Part model, mm, in its own coordinate system. A direction names the side the tool comes from. Give positions to 0.01 mm unless a question says otherwise; leave off trailing zeros. Order: outer loops, then holes, each group sorted by start corner. A loop starts at its lowest first (then second) coordinate and runs counter-clockwise, first axis right, second up. Notation, with made-up numbers: (85.5, 54) - (123.5, 54) arc R20 ccw to (123.5, 73) - close; hole circle Ø3 at (5.25, 41.25). An arc over 180 degrees is marked (long way). Use a Markdown table: item, result. Add a question column.
from build123d import *

# Parameters (mm, degrees)
BOSS_EXTRUDE1_DEPTH = 129


with BuildPart() as part:
    # Sketch1 → Boss-Extrude1 (new body)
    with BuildSketch(Plane.XY):
        with BuildLine():
            Line((-3.5, 4.403015152), (-3.5, 3.76))
            ThreePointArc((-3.5, 3.76), (-2.75, 3.01), (-3.5, 2.26))
            Line((-3.5, 2.26), (-3.5, 0.3))
            Line((-3.5, 0.3), (-3.2, 0))
            Line((-3.2, 0), (3.2, 0))
            Line((3.2, 0), (3.5, 0.3))
            Line((3.5, 0.3), (3.5, 2.26))
            ThreePointArc((3.5, 2.26), (2.75, 3.01), (3.5, 3.76))
            Line((3.5, 3.76), (3.5, 4.403015152))
            Line((3.5, 4.403015152), (3.203015152, 4.7))
            Line((3.203015152, 4.7), (-3.203015152, 4.7))
            Line((-3.203015152, 4.7), (-3.5, 4.403015152))
        make_face()
    extrude(amount=BOSS_EXTRUDE1_DEPTH)

    # Sketch2 → Cut-Revolve1 (revolve, cut)
    with BuildSketch(Plane(origin=(0, 0, 0), x_dir=(0, 0, -1), z_dir=(1, 0, 0)), mode=Mode.PRIVATE) as cut_revolve1_sk:
        Polygon((-4.5, 4.7), (-2.4, 4.7), (-2.4, 2.4), (-3.3, 2.4), (-3.3, 0), (-4.5, 0), align=None)
    revolve(cut_revolve1_sk.sketch.rotate(Axis((0, 0, 4.5), (0, 1, 0)), 180), axis=Axis((0, 0, 4.5), (0, 1, 0)), mode=Mode.SUBTRACT)

    # Sketch3 → Cut-Revolve2 (revolve, cut)
    with BuildSketch(Plane(origin=(0, 0, 0), x_dir=(0, 0, -1), z_dir=(1, 0, 0)), mode=Mode.PRIVATE) as cut_revolve2_sk:
        Polygon((-124.5, 4.7), (-122.4, 4.7), (-122.4, 2.4), (-123.3, 2.4), (-123.3, 0), (-124.5, 0), align=None)
    revolve(cut_revolve2_sk.sketch.rotate(Axis((0, 0, 124.5), (0, 1, 0)), 180), axis=Axis((0, 0, 124.5), (0, 1, 0)), mode=Mode.SUBTRACT)

    # Sketch4 → Cut-Revolve3 (revolve, cut)
    with BuildSketch(Plane(origin=(0, 0, 0), x_dir=(0, 0, -1), z_dir=(1, 0, 0)), mode=Mode.PRIVATE) as cut_revolve3_sk:
        Polygon((-109.5, 4.7), (-107.4, 4.7), (-107.4, 2.4), (-108.3, 2.4), (-108.3, 0), (-109.5, 0), align=None)
    revolve(cut_revolve3_sk.sketch.rotate(Axis((0, 0, 109.5), (0, 1, 0)), 180), axis=Axis((0, 0, 109.5), (0, 1, 0)), mode=Mode.SUBTRACT)

    # Sketch5 → Cut-Revolve4 (revolve, cut)
    with BuildSketch(Plane(origin=(0, 0, 0), x_dir=(0, 0, -1), z_dir=(1, 0, 0)), mode=Mode.PRIVATE) as cut_revolve4_sk:
        Polygon((-94.5, 4.7), (-92.4, 4.7), (-92.4, 2.4), (-93.3, 2.4), (-93.3, 0), (-94.5, 0), align=None)
    revolve(cut_revolve4_sk.sketch.rotate(Axis((0, 0, 94.5), (0, 1, 0)), 180), axis=Axis((0, 0, 94.5), (0, 1, 0)), mode=Mode.SUBTRACT)

    # Sketch6 → Cut-Revolve5 (revolve, cut)
    with BuildSketch(Plane(origin=(0, 0, 0), x_dir=(0, 0, -1), z_dir=(1, 0, 0)), mode=Mode.PRIVATE) as cut_revolve5_sk:
        Polygon((-79.5, 4.7), (-77.4, 4.7), (-77.4, 2.4), (-78.3, 2.4), (-78.3, 0), (-79.5, 0), align=None)
    revolve(cut_revolve5_sk.sketch.rotate(Axis((0, 0, 79.5), (0, 1, 0)), 180), axis=Axis((0, 0, 79.5), (0, 1, 0)), mode=Mode.SUBTRACT)

    # Sketch7 → Cut-Revolve6 (revolve, cut)
    with BuildSketch(Plane(origin=(0, 0, 0), x_dir=(0, 0, -1), z_dir=(1, 0, 0)), mode=Mode.PRIVATE) as cut_revolve6_sk:
        Polygon((-64.5, 4.7), (-62.4, 4.7), (-62.4, 2.4), (-63.3, 2.4), (-63.3, 0), (-64.5, 0), align=None)
    revolve(cut_revolve6_sk.sketch.rotate(Axis((0, 0, 64.5), (0, 1, 0)), 180), axis=Axis((0, 0, 64.5), (0, 1, 0)), mode=Mode.SUBTRACT)

    # Sketch8 → Cut-Revolve7 (revolve, cut)
    with BuildSketch(Plane(origin=(0, 0, 0), x_dir=(0, 0, -1), z_dir=(1, 0, 0)), mode=Mode.PRIVATE) as cut_revolve7_sk:
        Polygon((-49.5, 4.7), (-47.4, 4.7), (-47.4, 2.4), (-48.3, 2.4), (-48.3, 0), (-49.5, 0), align=None)
    revolve(cut_revolve7_sk.sketch.rotate(Axis((0, 0, 49.5), (0, 1, 0)), 180), axis=Axis((0, 0, 49.5), (0, 1, 0)), mode=Mode.SUBTRACT)

    # Sketch9 → Cut-Revolve8 (revolve, cut)
    with BuildSketch(Plane(origin=(0, 0, 0), x_dir=(0, 0, -1), z_dir=(1, 0, 0)), mode=Mode.PRIVATE) as cut_revolve8_sk:
        Polygon((-34.5, 4.7), (-32.4, 4.7), (-32.4, 2.4), (-33.3, 2.4), (-33.3, 0), (-34.5, 0), align=None)
    revolve(cut_revolve8_sk.sketch.rotate(Axis((0, 0, 34.5), (0, 1, 0)), 180), axis=Axis((0, 0, 34.5), (0, 1, 0)), mode=Mode.SUBTRACT)

    # Sketch10 → Cut-Revolve9 (revolve, cut)
    with BuildSketch(Plane(origin=(0, 0, 0), x_dir=(0, 0, -1), z_dir=(1, 0, 0)), mode=Mode.PRIVATE) as cut_revolve9_sk:
        Polygon((-19.5, 4.7), (-17.4, 4.7), (-17.4, 2.4), (-18.3, 2.4), (-18.3, 0), (-19.5, 0), align=None)
    revolve(cut_revolve9_sk.sketch.rotate(Axis((0, 0, 19.5), (0, 1, 0)), 180), axis=Axis((0, 0, 19.5), (0, 1, 0)), mode=Mode.SUBTRACT)


solid = part.part
1. Mould opens along Z. For faces 3 (the face through (-0.8, 3.53, 51.44)), 4 (the face through (-3.5, 1, 64)), 5 (the face through (0, 2, 0)) say: released by +Z, released by -Z, zero draft, split by the parting line, or undercut.
2. Drill centre lines: probe 1 along X at (y, z) = (0.55, 64.5); probe 2 along Y at (x, z) = (1, 78); probe 3 along Y at (x, z) = (3, 71). Where is each one in solid material? Low to high. Write a range as [from, to].
3. Cut at B-B (x = 0). State how many separate pieces and enclosed holes the cut face has, plus the area to 3 significant figures.
4. Cut at A-A (z = 64.5). Write the cut outline in (x, y).
5. Cut at C-C (z = 98.5). Write the cut outline in (x, y).
6. Pin check, flat tips, straight feed: P1, Ø3.5, axis at x = 0, z = 94.5, coming from the +Y side; P2, Ø2, axis at x = 0, z = 34.5, coming from the -Y side. Stop position of each tip, or through.
7. Tool access for faces 1 (the face through (-1.4, 2.4, 49.5)), 2 (the face through (0.05, 1.18, 93.3)): list every direction of +Z, -Z, +X, -X, +Y, -Y with a clear straight run to the whole face (end or side of a thin tool).
Responses:
| question | item | result |
|---|---|---|
| 1 | face 3 | undercut |
| 1 | face 4 | zero draft |
| 1 | face 5 | released by -Z |
| 2 | probe 1 | x = [-3.5, -1.2], [1.2, 3.5] |
| 2 | probe 2 | y = [0, 2.4] |
| 2 | probe 3 | y = [0, 2.45], [3.57, 4.7] |
| 3 | separate pieces | 10 |
| 3 | enclosed holes | 0 |
| 3 | area | 468 mm² |
| 4 | outline | (-3.5, 0.3) - (-3.2, 0) - (-1.2, 0) - (-1.2, 2.4) - (-2.1, 2.4) - (-2.1, 4.7) - (-3.2, 4.7) - (-3.5, 4.4) - (-3.5, 3.76) arc R0.75 cw to (-3.5, 2.26) - close; (1.2, 0) - (3.2, 0) - (3.5, 0.3) - (3.5, 2.26) arc R0.75 cw to (3.5, 3.76) - (3.5, 4.4) - (3.2, 4.7) - (2.1, 4.7) - (2.1, 2.4) - (1.2, 2.4) - close |
| 5 | outline | (-3.5, 0.3) - (-3.2, 0) - (3.2, 0) - (3.5, 0.3) - (3.5, 2.26) arc R0.75 cw to (3.5, 3.76) - (3.5, 4.4) - (3.2, 4.7) - (-3.2, 4.7) - (-3.5, 4.4) - (-3.5, 3.76) arc R0.75 cw to (-3.5, 2.26) - close |
| 6 | P1 | stops at y = 2.4 |
| 6 | P2 | passes through |
| 7 | face 1 | +Y |
| 7 | face 2 | +Y, -Y |
